```python
from build123d import *

# Parameters (mm, degrees)
F0_W     = 114.3
F0_H     = 50.8
F1_DEPTH = 50.8
F2_W     = 93.98
F2_H     = 17.78
F3_DEPTH = 38.1
F4_W     = 38.1
F4_H     = 17.78
F4_W_2   = 99.221253
F4_H_2   = 5.08
F5_DEPTH = 25.4
F6_DEPTH = 25.4


with BuildPart() as f1:
    # F0 (on Top) → F1 (new body)
    with BuildSketch(Plane.XY):
        with Locations((-0.874427, -22.725493)):
            Rectangle(F0_W, F0_H)
    extrude(amount=F1_DEPTH)

    # F2 (on face) → F3 (cut)
    with BuildSketch(Plane.XY.offset(50.8)):
        with Locations((-0.930555, -22.686988)):
            Rectangle(F2_W, F2_H)
    extrude(amount=-F3_DEPTH, mode=Mode.SUBTRACT)

    # F4 (on face) → F5 (cut)
    with BuildSketch(Plane.XZ.offset(48.125493)):
        with Locations((29.605573, 25.199144)):
            Rectangle(F4_W, F4_H)
        with Locations((-31.354427, 25.012475)):
            Rectangle(F4_W, F4_H)
        with Locations((-0.7938, 6.492384)):
            Rectangle(F4_W_2, F4_H_2)
    extrude(amount=-F5_DEPTH, mode=Mode.SUBTRACT)

    # F4 (on face) → F6 (cut)
    with BuildSketch(Plane.XZ.offset(48.125493)):
        with Locations((29.605573, 25.199144)):
            Rectangle(F4_W, F4_H)
        with Locations((-31.354427, 25.012475)):
            Rectangle(F4_W, F4_H)
        with Locations((-0.7938, 6.492384)):
            Rectangle(F4_W_2, F4_H_2)
    extrude(amount=-F6_DEPTH, mode=Mode.SUBTRACT)


solid = f1.part
```
Check sheet for the modelled part. Datum: model origin and axes. Units: mm. A direction names the side the tool comes from. Give positions to 0.01 mm unless a question says otherwise; leave off trailing zeros. Write each loop counter-clockwise with the first axis right and the second up, starting at its lowest first coordinate (ties: lowest second). Pieces come first, ordered by that corner, then holes.
Item 1: Cross-section at D-D (y = -33.5). Enter the section's corners in (x, z), and give its area (3 significant figures).
Item 2: Cross-section at B-B (x = -25). Enter the section's corners in (y, z), and give its area (3 significant figures).
Item 3: Cross-section at A-A (z = 30). Enter the section's corners in (x, y), and give its area (3 significant figures).
Item 4: Cross-section at C-C (z = 42). Enter the section's corners in (x, y), and give its area (3 significant figures).
Item 5: Scan lines: L1, parallel to Z at x = 35, y = -37; L2, parallel to Z at x = -35.5, y = -37; L3, parallel to X at y = -17, z = 34. Record each from-to range of solid material in increasing order.
Item 6: Access from +Z, -Z, +X, -X, +Y, -Y to the whole of each face (thin tool, end or side, straight path). Record for faces 5 (the face through (-2, 2.675, 25)), 6 (the face through (-2, -23, 12.7)), 7 (the face through (48.656, -36, 25)).
Item 7: Gauge pin test, flat ends, axial feed: pin 1 (3 mm diameter, centred on x = 39.5, y = -22.5, fed in from +Z); pin 2 (3 mm diameter, centred on x = 17, z = 32.5, fed in from -Y). Record the tip position at first contact, or that the pin passes through.
Item 8: Draft check along X on faces 1 (the face through (-58.024, -23, 25)), 2 (the face through (-2, -48.125, 25)), 3 (the face through (-2, -31.577, 36)), 4 (the face through (56.276, -23, 25)). Enter one of: released by +X, released by -X, zero draft, split by the parting line, or undercut.
Report:
1. outline: (-58.02, 0) - (56.28, 0) - (56.28, 50.8) - (-58.02, 50.8) - close; hole (-50.4, 3.95) - (48.82, 3.95) - (48.82, 9.03) - (-50.4, 9.03) - close; hole (-50.4, 16.12) - (-12.3, 16.12) - (-12.3, 33.9) - (-50.4, 33.9) - close; hole (10.56, 16.31) - (48.66, 16.31) - (48.66, 34.09) - (10.56, 34.09) - close
1. area: 3,950 mm2
2. outline: (-48.13, 0) - (2.67, 0) - (2.67, 50.8) - (-13.8, 50.8) - (-13.8, 12.7) - (-31.58, 12.7) - (-31.58, 16.12) - (-48.13, 16.12) - (-48.13, 9.03) - (-22.73, 9.03) - (-22.73, 3.95) - (-48.13, 3.95) - close; (-48.13, 33.9) - (-31.58, 33.9) - (-31.58, 50.8) - (-48.13, 50.8) - close
2. area: 1,480 mm2
3. outline: (-58.02, -48.13) - (-50.4, -48.13) - (-50.4, -22.73) - (-47.92, -22.73) - (-47.92, -13.8) - (46.06, -13.8) - (46.06, -22.73) - (48.66, -22.73) - (48.66, -48.13) - (56.28, -48.13) - (56.28, 2.67) - (-58.02, 2.67) - close; (-12.3, -48.13) - (10.56, -48.13) - (10.56, -31.58) - (-12.3, -31.58) - close
3. area: 2,830 mm2
4. outline: (-58.02, -48.13) - (56.28, -48.13) - (56.28, 2.67) - (-58.02, 2.67) - close; hole (-47.92, -31.58) - (46.06, -31.58) - (46.06, -13.8) - (-47.92, -13.8) - close
4. area: 4,140 mm2
5. L1: z = 0 to 3.95, 9.03 to 16.31, 34.09 to 50.8
5. L2: z = 0 to 3.95, 9.03 to 16.12, 33.9 to 50.8
5. L3: x = -58.02 to -47.92, 46.06 to 56.28
6. face 5: +Z, -Z, +X, -X, +Y
6. face 6: +Z
6. face 7: -Y
7. pin 1: stops at z = 12.7
7. pin 2: stops at y = -13.8
8. face 1: released by -X
8. face 2: zero draft
8. face 3: undercut
8. face 4: released by +X
